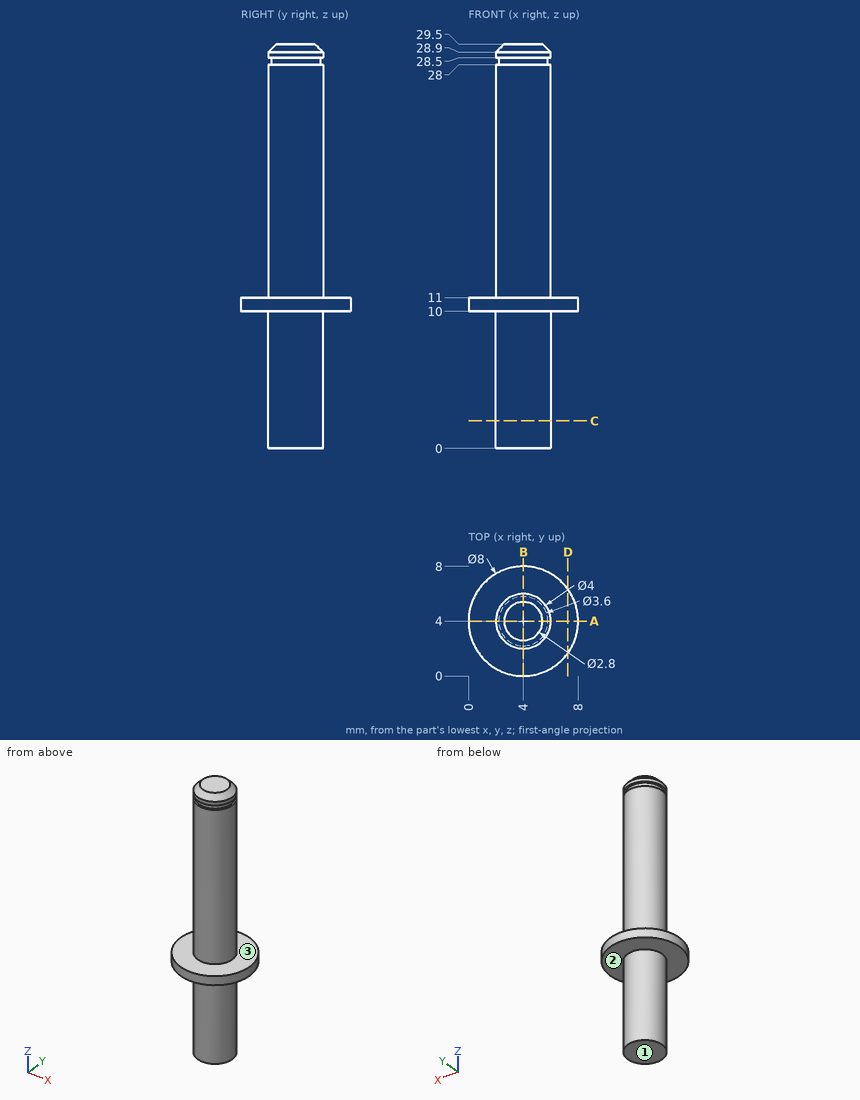
Check sheet for the drawn part. Datum: minimum x, y, z corner. Units: mm. A direction names the side the tool comes from. Round coordinates to 2 decimals unless told otherwise and drop trailing zeros. Order: outer loops, then holes, each group sorted by start corner. A loop starts at its lowest first (then second) coordinate and runs counter-clockwise, first axis right, second up. Notation, with made-up numbers: M 62.25,-36 L 111.25,-36 A13 ccw 111.25,-17 Z; hole C 1,49.5 d1. An arc over 180 degrees is marked long. Answer in a Markdown table with one row per item.
(1) Set-up check for the marked faces 1, 2 and 3: record each of +Z, -Z, +X, -X, +Y, -Y from which the full face is reachable in a straight line by a thin tool's end or side.
Findings:
| item | result |
|---|---|
| face 1 | -Z, +X, -X, +Y, -Y |
| face 2 | -Z |
| face 3 | +Z |
(2) Section check A-A on y = 4. Record the boundary of the cut face in (x, z).
Findings:
| item | result |
|---|---|
| outline | M 0,10 L 2,10 L 2,0 L 6,0 L 6,10 L 8,10 L 8,11 L 6,11 L 6,28 L 5.8,28 L 5.8,28.5 L 6,28.5 L 6,28.9 L 5.4,29.5 L 2.6,29.5 L 2,28.9 L 2,28.5 L 2.2,28.5 L 2.2,28 L 2,28 L 2,11 L 0,11 Z |
(3) Material ranges on line 1 along Z through (x, y) = (3.75, 7.25); line 2 along X through (y, z) = (2.25, 21.25); line 3 along Y through (x, z) = (2.75, 19), recorded low to high. Write a range as from..to.
Findings:
| item | result |
|---|---|
| line 1 | z = 10..11 |
| line 2 | x = 3.03..4.97 |
| line 3 | y = 2.44..5.56 |
(4) Gauge pin test, flat end, axial feed: pin 1 (2 mm diameter, centred on x = 2, z = 5.5, fed in from +Y). Record the tip position at first contact, or that the pin passes through.
Findings:
| item | result |
|---|---|
| pin 1 | stops at y = 5.73 |
(5) Section check C-C on z = 2. Record the boundary of the cut face in (x, y), plus the area to 3 significant figures.
Findings:
| item | result |
|---|---|
| outline | C 4,4 d4 |
| area | 12.6 mm^2 |
(6) Section check D-D on x = 7.25. Record the boundary of the cut face in (y, z).
Findings:
| item | result |
|---|---|
| outline | M 1.67,10 L 6.33,10 L 6.33,11 L 1.67,11 Z |
